Read the model definition and answer for the solid it produces. Units are mm, in the model's axes. A direction names the side the tool comes from. Coordinates: 2 decimals unless noted, no trailing zeros. Write each loop counter-clockwise with the first axis right and the second up, starting at its lowest first coordinate (ties: lowest second). Pieces come first, ordered by that corner, then holes.
1) The part is cut by section C-C (x = 81). Determine the outline of the cut face in (y, z), then the cut area to 3 significant figures.
2) Which of the six approach directions +Z, -Z, +X, -X, +Y, -Y give full straight-line access (tool end or side, diameter ignored) to faces 5 (the face through (-2.5, 3, -17.8)), 6 (the face through (10, 8, 0)), 7 (the face through (94.555, 64.077, -9.966)), 8 (the face through (94.18, 62.56, -9.97)), 9 (the face through (-2.3, 13.516, -3))?
3) Determine the mould class of faces 1 (the face through (68.569, 62.565, -9.966)), 2 (the face through (61.709, 30, -10)), 3 (the face through (81.75, 64.18, -9.97)), 4 (the face through (-1, 8, -9.95)) for opening direction Y: +Y half, -Y half, draft (parallel to the pull), parting line (faces both ways), or undercut.
4) The part is cut by section B-B (z = -19). Give the number of separate pieces and of enclosed holes in the cut face, then the cut area to 3 significant figures.
5) Find the intervals of material crossed by line 1 (X direction, y = 49.5, z = -15.5); line 2 (X direction, y = 27.5, z = -6); line 3 (Z direction, x = 14, y = 45), in increasing order.
6) The part is cut by section A-A (y = 25.5). Determine the outline of the cut face in (x, z), then the cut area to 3 significant figures.
7) Each of these flat-tipped pins is pushed along its axis until it touches: pin 1 Ø15.5 at (y, z) = (28, -3.5) entering from -X; pin 2 Ø8 at (y, z) = (52.5, -15) entering from -X; pin 3 Ø8 at (x, z) = (28, -20.5) entering from -Y. Where does it stop, or does it pass through?
from build123d import *

# Parameters (mm, degrees)
SKETCH1_W                  = 26.3
SKETCH1_H                  = 26.3
SKETCH1_W_2                = 20.3
SKETCH1_H_2                = 20.3
TUBE_EXTRUDE_DEPTH         = 60
HEX_EXTRUDE_DEPTH          = 26.3
SKETCH3_W                  = 23.3
SKETCH3_H                  = 26.968911086
TUBE_CENTER_CUT_DEPTH      = 1
TUBE_CENTER_CUT_DEPTH_BACK = 27.3
CUT_EXTRUDE1_START         = -3
CUT_EXTRUDE1_DEPTH         = 3
SKETCH5_W                  = 1
SKETCH5_H                  = 10.515544457
CUT_EXTRUDE2_DEPTH         = 27.3
FILLET1_R                  = 3
FILLET2_R                  = 1


with BuildPart() as part:
    # Sketch1 → Tube Extrude (new body)
    with BuildSketch(Plane(origin=(0, 0, 0), x_dir=(1, 0, 0), z_dir=(0, 1, 0))):
        with Locations((10.15, 10.15)):
            Rectangle(SKETCH1_W, SKETCH1_H)
        with Locations((10.15, 10.15)):
            Rectangle(SKETCH1_W_2, SKETCH1_H_2, mode=Mode.SUBTRACT)
    extrude(amount=TUBE_EXTRUDE_DEPTH)

    # Sketch2 → Hex Extrude (add)
    with BuildSketch(Plane.XY.offset(3)):
        Polygon((23.3, 15.649519053), (23.3, 0), (36.852881057, -7.824759526), (49.655762114, -0.433012702), (62.45864317, -7.824759526), (75.261524227, -0.433012702), (88.064405284, -7.824759526), (100.867286341, -0.433012702), (113.670167397, -7.824759526), (127.223048454, 0), (127.223048454, 15.649519053), (127.223048454, 44.350480947), (127.223048454, 60), (113.670167397, 67.824759526), (100.867286341, 60.433012702), (88.064405284, 67.824759526), (75.261524227, 60.433012702), (62.45864317, 67.824759526), (49.655762114, 60.433012702), (36.852881057, 67.824759526), (23.3, 60), (23.3, 44.350480947), align=None)
        Polygon((49.655762114, 16.082531755), (37.602881057, 23.041265877), (37.602881057, 36.958734123), (49.655762114, 43.917468245), (61.70864317, 36.958734123), (61.70864317, 23.041265877), align=None, mode=Mode.SUBTRACT)
        Polygon((36.102881057, 23.041265877), (24.8, 16.515544457), (24.8, 43.484455543), (36.102881057, 36.958734123), align=None, mode=Mode.SUBTRACT)
        Polygon((24.8, 0.866025404), (36.852881057, -6.092708719), (48.905762114, 0.866025404), (48.905762114, 14.783493649), (36.852881057, 21.742227772), (24.8, 14.783493649), align=None, mode=Mode.SUBTRACT)
        Polygon((50.405762114, 0.866025404), (62.45864317, -6.092708719), (74.511524227, 0.866025404), (74.511524227, 14.783493649), (62.45864317, 21.742227772), (50.405762114, 14.783493649), align=None, mode=Mode.SUBTRACT)
        Polygon((76.011524227, 0.866025404), (88.064405284, -6.092708719), (100.117286341, 0.866025404), (100.117286341, 14.783493649), (88.064405284, 21.742227772), (76.011524227, 14.783493649), align=None, mode=Mode.SUBTRACT)
        Polygon((125.723048454, 16.515544457), (114.420167397, 23.041265877), (114.420167397, 36.958734123), (125.723048454, 43.484455543), align=None, mode=Mode.SUBTRACT)
        Polygon((101.617286341, 0.866025404), (113.670167397, -6.092708719), (125.723048454, 0.866025404), (125.723048454, 14.783493649), (113.670167397, 21.742227772), (101.617286341, 14.783493649), align=None, mode=Mode.SUBTRACT)
        Polygon((24.8, 45.216506351), (36.852881057, 38.257772228), (48.905762114, 45.216506351), (48.905762114, 59.133974596), (36.852881057, 66.092708719), (24.8, 59.133974596), align=None, mode=Mode.SUBTRACT)
        Polygon((50.405762114, 45.216506351), (62.45864317, 38.257772228), (74.511524227, 45.216506351), (74.511524227, 59.133974596), (62.45864317, 66.092708719), (50.405762114, 59.133974596), align=None, mode=Mode.SUBTRACT)
        Polygon((76.011524227, 45.216506351), (88.064405284, 38.257772228), (100.117286341, 45.216506351), (100.117286341, 59.133974596), (88.064405284, 66.092708719), (76.011524227, 59.133974596), align=None, mode=Mode.SUBTRACT)
        Polygon((101.617286341, 45.216506351), (113.670167397, 38.257772228), (125.723048454, 45.216506351), (125.723048454, 59.133974596), (113.670167397, 66.092708719), (101.617286341, 59.133974596), align=None, mode=Mode.SUBTRACT)
        Polygon((75.261524227, 16.082531755), (87.314405284, 23.041265877), (87.314405284, 36.958734123), (75.261524227, 43.917468245), (63.20864317, 36.958734123), (63.20864317, 23.041265877), align=None, mode=Mode.SUBTRACT)
        Polygon((100.867286341, 16.082531755), (112.920167397, 23.041265877), (112.920167397, 36.958734123), (100.867286341, 43.917468245), (88.814405284, 36.958734123), (88.814405284, 23.041265877), align=None, mode=Mode.SUBTRACT)
    extrude(amount=-HEX_EXTRUDE_DEPTH)

    # Sketch3 → Tube Center Cut (cut, two sides)
    with BuildSketch(Plane.XY.offset(3)) as tube_center_cut_sk:
        with Locations((8.65, 30)):
            Rectangle(SKETCH3_W, SKETCH3_H)
    extrude(amount=TUBE_CENTER_CUT_DEPTH, mode=Mode.SUBTRACT)
    extrude(tube_center_cut_sk.sketch, amount=-TUBE_CENTER_CUT_DEPTH_BACK, mode=Mode.SUBTRACT)

    # Sketch4 → Cut-Extrude1 (cut)
    with BuildSketch(Plane.ZY.offset(3).offset(CUT_EXTRUDE1_START)):
        Polygon((-10.15, 60), (-10.35, 60), (-10.35, 0), (-10.15, 0), (-9.95, 0), (-9.95, 60), align=None)
    extrude(amount=CUT_EXTRUDE1_DEPTH, mode=Mode.SUBTRACT)

    # Sketch5 → Cut-Extrude2 (cut, through all)
    with BuildSketch(Plane.XY.offset(3)):
        with Locations((-2.5, 51.742227771)):
            Rectangle(SKETCH5_W, SKETCH5_H)
        with Locations((-2.5, 8.257772229)):
            Rectangle(SKETCH5_W, SKETCH5_H)
    extrude(amount=-CUT_EXTRUDE2_DEPTH, mode=Mode.SUBTRACT)

    # Fillet1
    fillet1_edges = [part.edges().sort_by_distance(p)[0] for p in [
        (-2, 51.742227772, -23.3),
        (-2, 51.742227772, 3),
        (-2, 8.257772228, -23.3),
        (-2, 8.257772228, 3),
        (24.8, 52.175240474, -23.3),
        (24.8, 52.175240474, 3),
        (24.8, 7.824759526, -23.3),
        (24.8, 7.824759526, 3),
        (24.8, 30, 3),
        (24.8, 30, -23.3),
    ]]
    fillet(fillet1_edges, radius=FILLET1_R)

    # Fillet2
    fillet2_edges = [part.edges().sort_by_distance(p)[0] for p in [
        (0, 0, -15.325),
        (10.15, 0, 0),
        (20.3, 0, -10.15),
        (10.15, 0, -20.3),
        (0, 60, -15.325),
        (10.15, 60, 0),
        (20.3, 60, -10.15),
        (10.15, 60, -20.3),
        (10.15, 43.484455543, -20.3),
        (10.15, 16.515544457, -20.3),
        (-3, 15.015544457, -23.3),
        (-3, 15.015544457, 3),
        (20.3, 30, 3),
        (10.15, 16.515544457, 0),
        (0, 16.515544457, -4.975),
        (0, 43.484455543, -15.325),
        (10.15, 43.484455543, 0),
        (20.3, 30, -23.3),
        (0, 43.484455543, -4.975),
        (0, 16.515544457, -15.325),
        (0, 60, -4.975),
        (0, 0, -4.975),
        (-3, 1.5, -23.3),
        (-3, 44.984455543, -23.3),
        (-3, 1.5, 3),
        (-3, 44.984455543, 3),
        (-3, 58.5, -23.3),
        (-3, 58.5, 3),
    ]]
    fillet(fillet2_edges, radius=FILLET2_R)


solid = part.part
Reported:
1. outline: (-3.75, -23.3) - (-2.01, -23.3) - (-2.01, 3) - (-3.75, 3) - close; (17.66, -23.3) - (19.4, -23.3) - (19.4, 3) - (17.66, 3) - close; (40.6, -23.3) - (42.34, -23.3) - (42.34, 3) - (40.6, 3) - close; (62.01, -23.3) - (63.75, -23.3) - (63.75, 3) - (62.01, 3) - close
1. area: 182 mm2
2. face 5: -Z, -X
2. face 6: +Y, -Y
2. face 7: +Z, -Z, +Y
2. face 8: +Z, -Z
2. face 9: +Z, -X
3. face 1: undercut
3. face 2: undercut
3. face 3: +Y half
3. face 4: draft
4. separate pieces: 3
4. enclosed holes: 13
4. area: 1,340 mm2
5. line 1: x = -2 to 0, 20.3 to 24.8, 48.91 to 50.41, 74.51 to 76.01, 100.12 to 101.62, 125.72 to 127.22
5. line 2: x = 20.3 to 24.8, 36.1 to 37.6, 61.71 to 63.21, 87.31 to 88.81, 112.92 to 114.42, 125.72 to 127.22
5. line 3: z = -23.3 to -20.3, 0 to 3
6. outline: (20.3, -22.3) arc R1 ccw to (21.3, -23.3) - (21.8, -23.3) arc R3 ccw to (24.8, -20.3) - (24.8, 0) arc R3 ccw to (21.8, 3) - (21.3, 3) arc R1 ccw to (20.3, 2) - close; (36.1, -23.3) - (37.6, -23.3) - (37.6, 3) - (36.1, 3) - close; (61.71, -23.3) - (63.21, -23.3) - (63.21, 3) - (61.71, 3) - close; (87.31, -23.3) - (88.81, -23.3) - (88.81, 3) - (87.31, 3) - close; (112.92, -23.3) - (114.42, -23.3) - (114.42, 3) - (112.92, 3) - close; (125.72, -23.3) - (127.22, -23.3) - (127.22, 3) - (125.72, 3) - close
6. area: 311 mm2
7. pin 1: stops at x = 20.3
7. pin 2: stops at x = -2
7. pin 3: stops at y = -5.02
